from build123d import *

# Parameters (mm, degrees)
SKETCH_W        = 10
SKETCH_H        = 17.5
SKETCH_R        = 2.5
PAD_DEPTH       = 7
SKETCH001_W     = 10
SKETCH001_H     = 6
POCKET_DEPTH    = 2
SKETCH002_R     = 1.1
POCKET001_DEPTH = 5.001
SKETCH003_R     = 4
PAD001_DEPTH    = 2
SKETCH004_R     = 2.5
POCKET002_DEPTH = 5
FILLET_R        = 4
FILLET001_R     = 1
FILLET002_R     = 1


with BuildPart() as part:
    # Sketch → Pad (new body)
    with BuildSketch(Plane.XY):
        with Locations((0, -3.75)):
            Rectangle(SKETCH_W, SKETCH_H)
        Circle(SKETCH_R, mode=Mode.SUBTRACT)
    extrude(amount=PAD_DEPTH)

    # Sketch001 (on Face6 of Pad) → Pocket (cut)
    with BuildSketch(Plane(origin=(0, 0, 0), x_dir=(1, 0, 0), z_dir=(0, 0, -1))):
        with Locations((0, 8)):
            Rectangle(SKETCH001_W, SKETCH001_H)
    extrude(amount=-POCKET_DEPTH, mode=Mode.SUBTRACT)

    # Sketch002 (on Face7 of Pocket) → Pocket001 (cut, through all)
    with BuildSketch(Plane(origin=(0, 0, 2), x_dir=(1, 0, 0), z_dir=(0, 0, -1))):
        with Locations((-1, 8)):
            Circle(SKETCH002_R)
    extrude(amount=-POCKET001_DEPTH, mode=Mode.SUBTRACT)

    # Sketch003 (on Face7 of Pad) → Pad001 (join)
    with BuildSketch(Plane.XY.offset(7)):
        Circle(SKETCH003_R)
    extrude(amount=PAD001_DEPTH)

    # Sketch004 (on Face15 of Pad001) → Pocket002 (cut)
    with BuildSketch(Plane.XY.offset(9)):
        Circle(SKETCH004_R)
    extrude(amount=-POCKET002_DEPTH, mode=Mode.SUBTRACT)

    # Fillet
    fillet_edges = [part.edges().sort_by_distance(p)[0] for p in [
        (5, 5, 3.5),
        (-5, 5, 3.5),
    ]]
    fillet(fillet_edges, radius=FILLET_R)

    # Fillet001
    fillet001_edges = [part.edges().sort_by_distance(p)[0] for p in [
        (-5, -12.5, 3.5),
    ]]
    fillet(fillet001_edges, radius=FILLET001_R)

    # Fillet002
    fillet002_edges = [part.edges().sort_by_distance(p)[0] for p in [
        (5, -12.5, 3.5),
    ]]
    fillet(fillet002_edges, radius=FILLET002_R)


solid = part.part
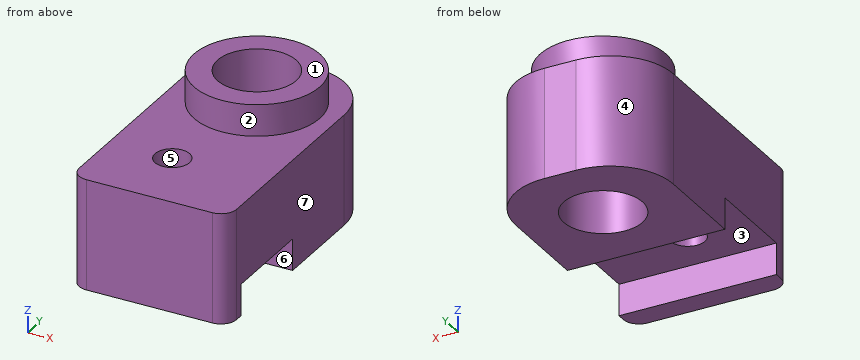
Design review of the part built by this model. Coordinates are the model's own, in mm. Face numbers are marked on the shaded views. A direction names the side the tool comes from. Round coordinates to 2 decimals unless told otherwise and drop trailing zeros. Write each loop counter-clockwise with the first axis right and the second up, starting at its lowest first coordinate (ties: lowest second). Pieces come first, ordered by that corner, then holes. Notation, with made-up numbers: (46.5, 60.5) -> (93.5, 60.5) arc R27 cw to (93.5, 97.5) -> close; hole circle Ø8 at (-15, 37.5). An arc over 180 degrees is marked (long way). One line per item, written item: value. Start each with the question number.
Q1. Add section A-A (y = 0). Give the boundary of the cut face in (x, z), then the cut area to 3 significant figures.
Q2. To check wall thickness, follow probe 1 along Y at (x, z) = (-1, 5.6); probe 2 along X at (y, z) = (-8, 5.1); probe 3 along Y at (x, z) = (0, 6). State the ranges of each line that lie inside material, in increasing order.
Q3. Add section B-B (z = 4). Give the boundary of the cut face in (x, y), then the cut area to 3 significant figures.
Q4. The part is to be moulded in two halves that separate along X. For the marked faces 4, 5, 6 and 7, say which applies: pulls with the +X half, pulls with the -X half, needs draft (parallel to the pull), parting line crosses it, or undercut.
Q5. Add section C-C (x = 2.25). Give the boundary of the cut face in (y, z), then the cut area to 3 significant figures.
Q6. Add section D-D (x = -1.75). Give the boundary of the cut face in (y, z), then the cut area to 3 significant figures.
Q7. Insertion check: P1, Ø1.8, axis at x = 2.5, y = -8, coming from the -Z side. The pin has a flat end and moves straight along its axis. Give the tip position at first contact, or say it passes through.
Q8. Tool access review of the marked faces 1, 2 and 3: name each direction out of +Z, -Z, +X, -X, +Y, -Y from which nothing blocks a thin tool from reaching the whole face with its end or side.
Response:
1. outline: (-5, 0) -> (-2.5, 0) -> (-2.5, 9) -> (-4, 9) -> (-4, 7) -> (-5, 7) -> close; (2.5, 0) -> (5, 0) -> (5, 7) -> (4, 7) -> (4, 9) -> (2.5, 9) -> close
1. area: 41.0 mm^2
2. probe 1: y = -12.5 to -9.1, -6.9 to -2.29, 2.29 to 5
2. probe 2: x = -5 to -2.1, 0.1 to 5
2. probe 3: y = -12.5 to -8.46, -7.54 to -2.5, 2.5 to 5
3. outline: (-5, -11.5) arc R1 ccw to (-4, -12.5) -> (4, -12.5) arc R1 ccw to (5, -11.5) -> (5, 1) arc R4 ccw to (1, 5) -> (-1, 5) arc R4 ccw to (-5, 1) -> close; hole circle Ø5 at (0, 0); hole circle Ø2.2 at (-1, -8)
3. area: 144 mm^2
4. face 4: pulls with the -X half
4. face 5: undercut
4. face 6: needs draft
4. face 7: pulls with the +X half
5. outline: (-12.5, 0) -> (-11, 0) -> (-11, 2) -> (-5, 2) -> (-5, 0) -> (-1.09, 0) -> (-1.09, 9) -> (-3.31, 9) -> (-3.31, 7) -> (-12.5, 7) -> close; (1.09, 0) -> (4.8, 0) -> (4.8, 7) -> (3.31, 7) -> (3.31, 9) -> (1.09, 9) -> close
5. area: 103 mm^2
6. outline: (-12.5, 0) -> (-11, 0) -> (-11, 2) -> (-8.8, 2) -> (-8.8, 7) -> (-12.5, 7) -> close; (-7.2, 2) -> (-5, 2) -> (-5, 0) -> (-1.79, 0) -> (-1.79, 9) -> (-3.6, 9) -> (-3.6, 7) -> (-7.2, 7) -> close; (1.79, 0) -> (4.93, 0) -> (4.93, 7) -> (3.6, 7) -> (3.6, 9) -> (1.79, 9) -> close
6. area: 84.2 mm^2
7. P1: stops at z = 2
8. face 1: +Z, +X, -X, +Y, -Y
8. face 2: +Z
8. face 3: -Z, +X, -X
